For this review, take the finished solid that the model builds, in its own axes (mm). Face numbers are marked on the shaded views. Coordinates: 2 decimals unless noted, no trailing zeros. Order: outer loops, then holes, each group sorted by start corner. A loop starts at its lowest first (then second) coordinate and runs counter-clockwise, first axis right, second up.
from build123d import *

# Parameters (mm, degrees)
BOSS_EXTRUDE1_DEPTH = 5
BOSS_EXTRUDE2_DEPTH = 165
SKETCH3_R           = 1.5
CUT_EXTRUDE1_DEPTH  = 165
SKETCH4_R           = 1.5
CUT_EXTRUDE2_DEPTH  = 3
CHAMFER1_SIZE       = 1


with BuildPart() as part:
    # Sketch1 → Boss-Extrude1 (new body)
    with BuildSketch(Plane.XY):
        with BuildLine():
            Line((269.472126518, 195.948380571), (259.892978717, 190.352443674))
            ThreePointArc((259.892978717, 190.352443674), (259.523120334, 189.974415309), (259.397797004, 189.460611133))
            Line((259.397797004, 189.460611133), (259.926827069, 170.821662041))
            ThreePointArc((259.926827069, 170.821662041), (260.081091813, 170.315793424), (260.471796679, 169.959352158))
            Line((260.471796679, 169.959352158), (270.352926754, 164.915757134))
            ThreePointArc((270.352926754, 164.915757134), (270.835926205, 164.806841188), (271.311970321, 164.942977708))
            Line((271.311970321, 164.942977708), (280.891118122, 170.538914605))
            ThreePointArc((280.891118122, 170.538914605), (281.260976505, 170.916942969), (281.386299835, 171.430747146))
            Line((281.386299835, 171.430747146), (280.85726977, 190.069696238))
            ThreePointArc((280.85726977, 190.069696238), (280.703005026, 190.575564854), (280.31230016, 190.93200612))
            Line((280.31230016, 190.93200612), (270.431170085, 195.975601144))
            ThreePointArc((270.431170085, 195.975601144), (269.948170634, 196.08451709), (269.472126518, 195.948380571))
        make_face()
        with BuildLine():
            Line((269.536796739, 193.669899558), (262.417863464, 189.511168301))
            ThreePointArc((262.417863464, 189.511168301), (262.048005081, 189.133139936), (261.922681752, 188.61933576))
            Line((261.922681752, 188.61933576), (262.399929545, 171.804795492))
            ThreePointArc((262.399929545, 171.804795492), (262.554194289, 171.298926876), (262.944899155, 170.942485609))
            Line((262.944899155, 170.942485609), (270.288256533, 167.194238147))
            ThreePointArc((270.288256533, 167.194238147), (270.771255984, 167.085322201), (271.2473001, 167.22145872))
            Line((271.2473001, 167.22145872), (278.366233375, 171.380189978))
            ThreePointArc((278.366233375, 171.380189978), (278.736091758, 171.758218342), (278.861415087, 172.272022518))
            Line((278.861415087, 172.272022518), (278.384167294, 189.086562786))
            ThreePointArc((278.384167294, 189.086562786), (278.22990255, 189.592431403), (277.839197684, 189.948872669))
            Line((277.839197684, 189.948872669), (270.495840306, 193.697120131))
            ThreePointArc((270.495840306, 193.697120131), (270.012840855, 193.806036078), (269.536796739, 193.669899558))
        make_face(mode=Mode.SUBTRACT)
    extrude(amount=BOSS_EXTRUDE1_DEPTH)

    # Sketch2 → Boss-Extrude2 (add)
    with BuildSketch(Plane.XY.offset(5)):
        Polygon((279.857672325, 190.041324622), (269.97654225, 195.084919646), (260.397394449, 189.488982749), (260.926424514, 170.850033657), (270.807554589, 165.806438633), (280.38670239, 171.40237553), align=None)
        with BuildLine():
            Line((269.536796739, 193.669899558), (262.417863464, 189.511168301))
            ThreePointArc((262.417863464, 189.511168301), (262.048005081, 189.133139936), (261.922681752, 188.61933576))
            Line((261.922681752, 188.61933576), (262.399929545, 171.804795492))
            ThreePointArc((262.399929545, 171.804795492), (262.554194289, 171.298926876), (262.944899155, 170.942485609))
            Line((262.944899155, 170.942485609), (270.288256533, 167.194238147))
            ThreePointArc((270.288256533, 167.194238147), (270.771255984, 167.085322201), (271.2473001, 167.22145872))
            Line((271.2473001, 167.22145872), (278.366233375, 171.380189978))
            ThreePointArc((278.366233375, 171.380189978), (278.736091758, 171.758218342), (278.861415087, 172.272022518))
            Line((278.861415087, 172.272022518), (278.384167294, 189.086562786))
            ThreePointArc((278.384167294, 189.086562786), (278.22990255, 189.592431403), (277.839197684, 189.948872669))
            Line((277.839197684, 189.948872669), (270.495840306, 193.697120131))
            ThreePointArc((270.495840306, 193.697120131), (270.012840855, 193.806036078), (269.536796739, 193.669899558))
        make_face(mode=Mode.SUBTRACT)
    extrude(amount=BOSS_EXTRUDE2_DEPTH)

    # Sketch3 → Cut-Extrude1 (cut)
    with BuildSketch(Plane(origin=(265.561732352, 7.537449653, 0), x_dir=(0, 0, 1), z_dir=(-0.999597445, -0.028371616, 0))):
        with Locations((107, 176.701580488)):
            Circle(SKETCH3_R)
        with Locations((107, 168.701580488)):
            Circle(SKETCH3_R)
        with Locations((125, 176.701580488)):
            Circle(SKETCH3_R)
        with Locations((125, 168.701580488)):
            Circle(SKETCH3_R)
        Polygon((170, 187.346716472), (170, 158.056444505), (141, 158.056444505), align=None)
    extrude(amount=-CUT_EXTRUDE1_DEPTH, mode=Mode.SUBTRACT)

    # Sketch4 → Cut-Extrude2 (cut)
    with BuildSketch(Plane(origin=(265.561732352, 7.537449653, 0), x_dir=(0, 0, 1), z_dir=(-0.999597445, -0.028371616, 0))):
        with Locations((15, 172.701580488)):
            Circle(SKETCH4_R)
    extrude(amount=-CUT_EXTRUDE2_DEPTH, mode=Mode.SUBTRACT)

    # Chamfer1
    chamfer1_edges = [part.edges().sort_by_distance(p)[0] for p in [
        (262.274792111, 176.213675847, 105.5),
        (278.736277653, 176.680902874, 105.5),
        (262.047819186, 184.210455405, 123.5),
        (278.509304728, 184.677682431, 123.5),
        (262.274792111, 176.213675847, 123.5),
        (278.736277653, 176.680902874, 123.5),
        (262.047819186, 184.210455405, 105.5),
        (278.509304728, 184.677682431, 105.5),
        (262.161305648, 180.212065626, 13.5),
    ]]
    chamfer(chamfer1_edges, length=CHAMFER1_SIZE)


solid = part.part
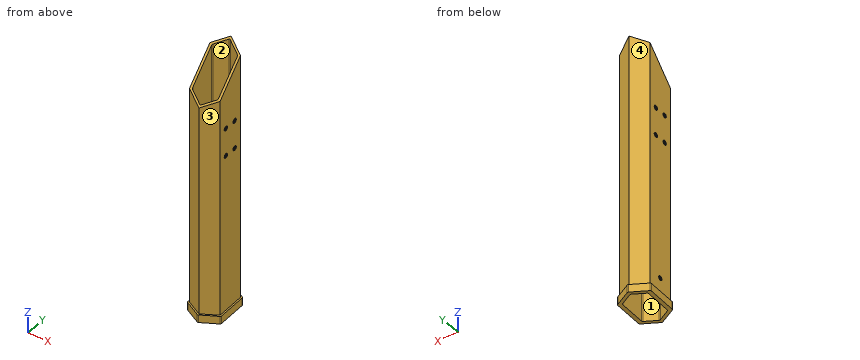
1. Take a section at C-C, the plane z = 156.5. Give the boundary of the cut face in (x, y).
Answer below:
outline: (260.4, 189.49) - (260.63, 181.18) - (262.13, 181.22) - (261.92, 188.62) arc R1 cw to (262.42, 189.51) - (269.54, 193.67) arc R1 cw to (270.5, 193.7) - (277.84, 189.95) arc R1 cw to (278.38, 189.09) - (278.59, 181.69) - (280.09, 181.73) - (279.86, 190.04) - (269.98, 195.08) - close
2. Take a section at B-B, the plane x = 265. Give the boundary of the cut face in (y, z).
Answer below:
outline: (167.65, 0) - (169.89, 0) - (169.89, 145.21) - (168.77, 144.1) - (168.77, 5) - (167.65, 5) - close; (191.02, 0) - (193.34, 0) - (193.34, 5) - (192.18, 5) - (192.18, 167.26) - (191.02, 166.12) - close
3. Take a section at D-D, the plane x = 276. Give the boundary of the cut face in (y, z), plus the area to 3 significant figures.
Answer below:
outline: (167.68, 0) - (170, 0) - (170, 145) - (168.84, 143.86) - (168.84, 5) - (167.68, 5) - close; (190.89, 0) - (193.13, 0) - (193.13, 5) - (192.01, 5) - (192.01, 166.79) - (190.89, 165.68) - close
area: 365 mm2
4. Take a section at A-A, the plane z = 46. Give the boundary of the cut face in (x, y), plus the area to 3 significant figures.
Answer below:
outline: (260.4, 189.49) - (260.93, 170.85) - (270.81, 165.81) - (280.39, 171.4) - (279.86, 190.04) - (269.98, 195.08) - close; hole (261.92, 188.62) - (262.4, 171.8) arc R1 ccw to (262.94, 170.94) - (270.29, 167.19) arc R1 ccw to (271.25, 167.22) - (278.37, 171.38) arc R1 ccw to (278.86, 172.27) - (278.38, 189.09) arc R1 ccw to (277.84, 189.95) - (270.5, 193.7) arc R1 ccw to (269.54, 193.67) - (262.42, 189.51) arc R1 ccw to start
area: 96.3 mm2
5. The part is to be moulded in two halves that separate along X. For the marked faces 1, 2, 3 and 4, say which applies: +X half, -X half, draft (parallel to the pull), parting line (faces both ways), or undercut.
Answer below:
face 1: undercut
face 2: undercut
face 3: +X half
face 4: -X half
6. Clearance check with flat-ended pins moving along their axes: pin 1 Ø1 at (x, z) = (273, 58.5) entering from -Y; pin 2 Ø12 at (x, y) = (275, 189) entering from -Z; pin 3 Ø4 at (y, z) = (186.5, 74.5) entering from +X; pin 4 Ø6 at (y, z) = (180, 38.5) entering from -X. State where each tip first meets the part, or that it passes through.
Answer below:
pin 1: stops at y = 166.8
pin 2: stops at z = 0
pin 3: stops at x = 280.01
pin 4: stops at x = 260.58
7. To check wall thickness, follow L1, parallel to X at y = 191, z = 67.5; L2, parallel to X at y = 188, z = 90 (3 decimals); L3, parallel to Y at x = 269.75, z = 119. State the ranges of each line that lie inside material, in increasing order.
Answer below:
L1: x = 262.98 to 264.97, 275.78 to 277.98
L2: x = 260.44 to 261.94, 278.415 to 279.916
L3: y = 166.35 to 167.47, 193.76 to 194.95
